Solid Edge part; units mm, degrees
sketch "Sketch1" plane through (0, 0, 0) normal (0, 0, 1) x (1, 0, 0)
  line L0 (-37.2884, 10.9984) -> (-27.5384, 10.9984)
  line L1 (-27.5384, 10.9984) -> (-27.5384, 20.7484)
  line L2 (-27.5384, 20.7484) -> (-37.2884, 20.7484)
  line L3 (-37.2884, 20.7484) -> (-37.2884, 10.9984)
  dimension "D1" = 27.5384
  dimension "D2" = 37.2884
extrude "Protrusion1" add sketch "Sketch1" along normal blind 25
sketch "Sketch2" plane through (-32.5384, 13.9984, 12.5) normal (0, -1, 0) x (0, 0, 1)
  line L0 (12.5, 4.75) -> (9.2, 4.75)
  line L1 (9.2, 4.75) -> (9.2, 6.25)
  line L2 (9.2, 6.25) -> (12.5, 4.75)
extrude "ExtrudedProtrusion_3" add sketch "Sketch2" against normal blind 3.5
sketch "Sketch3" plane through (-32.5384, 17.4984, 0) normal (0, 0, -1) x (0, 1, 0)
  line L0 (4.25, -3.75) -> (4.25, -5.75)
  line L1 (4.25, -5.75) -> (2.25, -5.75)
  line L2 (2.25, -3.75) -> (2.25, -5.75)
  line L3 (4.25, -3.75) -> (2.25, -3.75)
  line L4 (-5.5, -5.5) -> (-7.5, -5.5)
  line L5 (-7.5, -5.5) -> (-7.5, -3.5)
  line L6 (-5.5, -3.5) -> (-7.5, -3.5)
  line L7 (-5.5, -3.5) -> (-5.5, -5.5)
  line L8 (-7.5, 4) -> (-7.5, 6)
  line L9 (-7.5, 6) -> (-5.5, 6)
  line L10 (-5.5, 6) -> (-5.5, 4)
  line L11 (-7.5, 4) -> (-5.5, 4)
  line L12 (2.25, 6) -> (4.25, 6)
  line L13 (4.25, 6) -> (4.25, 4)
  line L14 (2.25, 4) -> (4.25, 4)
  line L15 (2.25, 6) -> (2.25, 4)
  dimension "D1" = 7.5
  dimension "D2" = 5.5
  dimension "D3" = 2.25
extrude "ExtrudedProtrusion_4" add sketch "Sketch3" against normal blind 12
sketch "Sketch4" plane through (-32.2884, 17.4984, 12.5) normal (1, 0, 0) x (0, -1, 0)
  line L0 (6.5, 9.25) -> (8.75, 9.25)
  line L1 (8.75, 9.25) -> (8.75, -1.4212)
  line L2 (10.5, -2.3314) -> (8.75, -1.4212)
  line L3 (10.5, -2.3314) -> (10.5, -2.9)
  line L4 (10.5, -2.9) -> (7.5, -8.25)
  line L5 (7.5, 6.75) -> (7.5, -8.25)
  line L6 (6.5, 6.75) -> (7.5, 6.75)
  line L7 (6.5, 9.25) -> (6.5, 6.75)
  line L8 (-3.25, 9.25) -> (-5.5, 9.25)
  line L9 (-5.5, 9.25) -> (-5.5, -1.4212)
  line L10 (-7.25, -2.3314) -> (-5.5, -1.4212)
  line L11 (-7.25, -2.3314) -> (-7.25, -2.9)
  line L12 (-7.25, -2.9) -> (-4.25, -8.25)
  line L13 (-4.25, 6.75) -> (-4.25, -8.25)
  line L14 (-3.25, 6.75) -> (-4.25, 6.75)
  line L15 (-3.25, 9.25) -> (-3.25, 6.75)
extrude "ExtrudedProtrusion_5" add sketch "Sketch4" along normal mid plane 5
sketch "Sketch5" plane through (-32.5384, 17.4984, 25) normal (0, 0, 1) x (0, 1, 0)
  line L0 (-1, -0.75) -> (2.5, -0.75)
  line L1 (2.5, -0.75) -> (2.5, -4.25)
  line L2 (2.5, -4.25) -> (-1, -4.25)
  line L3 (-1, -4.25) -> (-1, -0.75)
  line L4 (-1, 3.9418) -> (2.5, 3.9418)
  line L5 (2.5, 3.9418) -> (2.5, 1.4418)
  line L6 (2.5, 1.4418) -> (1.5, 0.4418)
  line L7 (1.5, 0.4418) -> (0, 0.4418)
  line L8 (0, 0.4418) -> (-1, 1.4418)
  line L9 (-1, 1.4418) -> (-1, 3.9418)
  line L10 (-5.5, 3.9418) -> (-2, 3.9418)
  line L11 (-2, 3.9418) -> (-2, 0.4418)
  line L12 (-2, 0.4418) -> (-5.5, 0.4418)
  line L13 (-5.5, 0.4418) -> (-5.5, 3.9418)
  line L14 (-5.5, -0.75) -> (-2, -0.75)
  line L15 (-2, -0.75) -> (-2, -3.25)
  line L16 (-2, -3.25) -> (-3, -4.25)
  line L17 (-3, -4.25) -> (-4.5, -4.25)
  line L18 (-4.5, -4.25) -> (-5.5, -3.25)
  line L19 (-5.5, -3.25) -> (-5.5, -0.75)
  dimension "D1" = 2
  dimension "D2" = 1
  dimension "D3" = 2.5
  dimension "D4" = 2.5
  dimension "D5" = 2
extrude "ExtrudedCutout_1" cut sketch "Sketch5" against normal blind 9
sketch "Sketch6" plane through (-32.5384, 17.4984, 0) normal (0, 0, -1) x (-1, 0, 0)
  line L0 (3.9419, -2) -> (0.4419, -2)
  line L1 (0.4419, -2) -> (0.4419, -5.5)
  line L2 (0.4419, -5.5) -> (3.9419, -5.5)
  line L3 (3.9419, -5.5) -> (3.9419, -2)
  line L4 (-0.75, -2) -> (-4.25, -2)
  line L5 (-4.25, -2) -> (-4.25, -5.5)
  line L6 (-4.25, -5.5) -> (-0.75, -5.5)
  line L7 (-0.75, -5.5) -> (-0.75, -2)
  line L8 (-0.75, 2.5) -> (-4.25, 2.5)
  line L9 (-4.25, 2.5) -> (-4.25, -1)
  line L10 (-4.25, -1) -> (-0.75, -1)
  line L11 (-0.75, -1) -> (-0.75, 2.5)
  line L12 (3.9419, 2.5) -> (0.4419, 2.5)
  line L13 (0.4419, 2.5) -> (0.4419, -1)
  line L14 (0.4419, -1) -> (3.9419, -1)
  line L15 (3.9419, -1) -> (3.9419, 2.5)
extrude "ExtrudedCutout_2" cut sketch "Sketch6" against normal blind 6
sketch "Sketch7" plane through (-34.7303, 13.7484, 6) normal (0, 0, -1) x (1, 0, 0)
  circle A0 centre (0, 0) radius 1
  circle A1 centre (4.6919, 0) radius 1
  circle A2 centre (4.6919, -4.5) radius 1
  circle A3 centre (-0.0581, -4.5) radius 1
extrude "Cutout1" cut sketch "Sketch7" against normal through all
Geometry: final body of the model. Coordinates: model frame, mm. A direction names the side the tool comes from. Round coordinates to 2 decimals unless told otherwise and drop trailing zeros. Write each loop counter-clockwise with the first axis right and the second up, starting at its lowest first coordinate (ties: lowest second). Pieces come first, ordered by that corner, then holes.
Item 1: Set-up query: faces 4 (the face through (-31, 15, 16)), 5 (the face through (-35, 15, 6)), 6 (the face through (-28, 21.748, 6)). Return all of +Z, -Z, +X, -X, +Y, -Y with unobstructed straight access to the full face (end or side cutting, diameter ignored); none if empty.
Item 2: Mould query, pull axis X, two halves, no side actions, for faces 1 (the face through (-32.32, 8.48, 18.04)), 2 (the face through (-28.781, 12.505, 20.563)), 3 (the face through (-38.038, 11, 6)). Classes: +X half, -X half, draft (parallel to the pull), parting line (faces both ways), or undercut.
Item 3: Section query C-C (z = 21.25). Return loops of the section in (x, y), plus the area to 3 significant figures.
Item 4: Pin query (flat end, axial travel): P1, Ø1.2, axis at y = 9.5, z = 13, coming from the -X side; P2, Ø3, axis at x = -36, z = 22.5, coming from the +Y side; P3, Ø3, axis at x = -35.5, z = 19.5, coming from the -Y side. Return the tip coordinate at first contact, or that it passes through.
Item 5: Section query B-B (x = -32.25). Return loops of the section in (y, z), plus the area to 3 significant figures.
Item 6: Material intervals for L1, parallel to X at y = 13, z = 1.5; L2, parallel to X at y = 18.25, z = 13.5; L3, parallel to Y at x = -30.5, z = 22.25, sorted ascending.
Item 7: Section query A-A (z = 9.75). Give the number of separate pieces and of enclosed holes in the cut face, plus the area to 3 significant figures.
Completed:
1. face 4: +Z
1. face 5: -Z
1. face 6: +Z, -Z, +X, +Y
2. face 1: draft
2. face 2: undercut
2. face 3: -X half
3. outline: (-37.29, 11) - (-27.54, 11) - (-27.54, 20.75) - (-37.29, 20.75) - close; hole (-36.48, 12) - (-32.98, 12) - (-32.98, 15.5) - (-36.48, 15.5) - close; hole (-36.48, 16.5) - (-33.98, 16.5) - (-32.98, 17.5) - (-32.98, 19) - (-33.98, 20) - (-36.48, 20) - close; hole (-31.79, 12) - (-29.29, 12) - (-28.29, 13) - (-28.29, 14.5) - (-29.29, 15.5) - (-31.79, 15.5) - close; hole (-31.79, 16.5) - (-28.29, 16.5) - (-28.29, 20) - (-31.79, 20) - close
3. area: 48.1 mm2
4. P1: stops at x = -34.79
4. P2: stops at y = 20.75
4. P3: stops at y = 8.56
5. outline: (7, 14.83) - (8.75, 13.92) - (8.75, 3.25) - (11, 3.25) - (11, 0) - (20.75, 0) - (20.75, 3.25) - (23, 3.25) - (23, 13.92) - (24.75, 14.83) - (24.75, 15.4) - (21.75, 20.75) - (21.75, 5.75) - (20.75, 5.75) - (20.75, 25) - (11, 25) - (11, 5.75) - (10, 5.75) - (10, 20.75) - (7, 15.4) - close
5. area: 299 mm2
6. L1: x = -37.29 to -36.48, -32.98 to -31.79, -28.29 to -27.54
6. L2: x = -37.29 to -35.79, -33.79 to -31.04, -29.04 to -27.54
6. L3: y = 11 to 12, 15.5 to 16.5, 20 to 20.75
7. separate pieces: 3
7. enclosed holes: 4
7. area: 107 mm2
